Verification items for the finished model (mm, model axes). Round coordinates to 2 decimals unless told otherwise and drop trailing zeros. Loops run counter-clockwise (first coordinate to the right, second up) from the corner with the lowest first, then second, coordinate; pieces in that order, holes last. Notation, with made-up numbers: (37, 4.25) - (45, 4.25) arc R15 cw to (45, 23.25) - close; hole circle Ø6 at (4.5, -18.5). An arc over 180 degrees is marked (long way). Use CSV: the item, a comma, the result in double quotes.
```python
from build123d import *

# Parameters (mm, degrees)
SKETCH_1_W                  = 145
SKETCH_1_H                  = 80
EXTRUDE_1_DEPTH             = 2
SKETCH_2_R                  = 1.5
CUT_EXTRUDE_1_DEPTH         = 2
PATTERN_LINEAR_1_COUNT      = 2
PATTERN_LINEAR_1_PITCH      = 137
PATTERN_LINEAR_1_COUNT_DIR2 = 2
PATTERN_LINEAR_1_PITCH_DIR2 = 72


with BuildPart() as part:
    # Эскиз1 → Бобышка-Вытянуть1 (new body)
    with BuildSketch(Plane.XY):
        with Locations((72.5, 40)):
            Rectangle(SKETCH_1_W, SKETCH_1_H)
    extrude(amount=EXTRUDE_1_DEPTH)

    # Эскиз2 → Вырез-Вытянуть1 (cut)
    with BuildSketch(Plane.XY.offset(2)):
        with Locations((4, 76)):
            Circle(SKETCH_2_R)
    cut_extrude_1 = extrude(amount=-CUT_EXTRUDE_1_DEPTH, mode=Mode.SUBTRACT)

    # Линейный массив1: Cut-Extrude 1 2 × 2
    with Locations(*[(i * PATTERN_LINEAR_1_PITCH, -j * PATTERN_LINEAR_1_PITCH_DIR2, 0) for i in range(PATTERN_LINEAR_1_COUNT) for j in range(PATTERN_LINEAR_1_COUNT_DIR2) if (i, j) != (0, 0)]):
        add(cut_extrude_1, mode=Mode.SUBTRACT)


solid = part.part
```
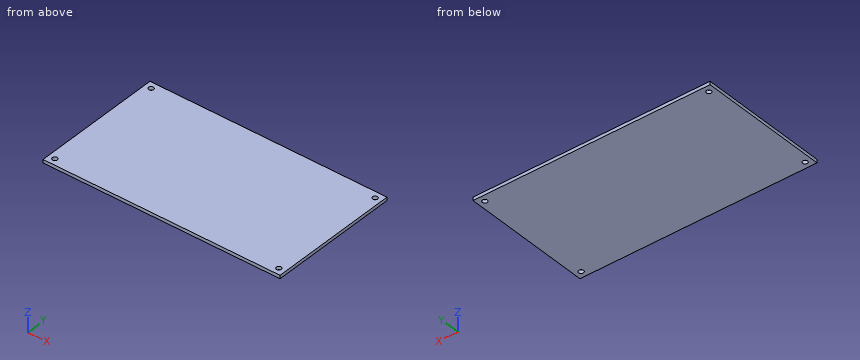
1) Cross-section at A-A, the plane y = 76. Record the cut outline in (x, z).
Returned:
outline,"(0, 0) - (2.5, 0) - (2.5, 2) - (0, 2) - close; (5.5, 0) - (139.5, 0) - (139.5, 2) - (5.5, 2) - close; (142.5, 0) - (145, 0) - (145, 2) - (142.5, 2) - close"
2) Cross-section at B-B, the plane x = 4. Record the cut outline in (y, z), then the cut area to 3 significant figures.
Returned:
outline,"(0, 0) - (2.5, 0) - (2.5, 2) - (0, 2) - close; (5.5, 0) - (74.5, 0) - (74.5, 2) - (5.5, 2) - close; (77.5, 0) - (80, 0) - (80, 2) - (77.5, 2) - close"
area,"148 mm²"
3) Gauge pin test, flat end, axial feed: pin 1 Ø2.5 at (x, y) = (141, 76) entering from +Z. Record the tip position at first contact, or that the pin passes through.
Returned:
pin 1,"passes through"
4) Thickness scan on probe 1 along X at (y, z) = (76, 1.5); probe 2 along Y at (x, z) = (4, 1.2). Record the ranges inside material, lowest first. Write a range as [from, to].
Returned:
probe 1,"x = [0, 2.5], [5.5, 139.5], [142.5, 145]"
probe 2,"y = [0, 2.5], [5.5, 74.5], [77.5, 80]"
